Autodesk Inventor part; units mm, degrees
ref_plane "YZ Plane" through (0, 0, 0) normal (1, 0, 0) x (0, 1, 0)
ref_plane "XZ Plane" through (0, 0, 0) normal (0, 1, 0) x (-1, 0, 0)
ref_plane "XY Plane" through (0, 0, 0) normal (0, 0, 1) x (1, 0, 0)
sketch "Skizze1" plane through (0, 0, 0) normal (0, 0, 1) x (1, 0, 0)
  line L0 (-20, 20) -> (20, 20)
  line L1 (20, 20) -> (20, -20)
  line L2 (20, -20) -> (-20, -20)
  line L3 (-20, -20) -> (-20, 20)
  line L4 (0, 20) -> (0, -20)
  line L5 (-20, 0) -> (20, 0)
  point P0 (0, 0)
  point P1 (0, 0)
  point P2 (-20, 0)
  point P3 (0, 0)
  point P4 (20, 0)
  dimension "d1" = 40
  dimension "d2" = 40
extrude "Extrusion1" add sketch "Skizze1" along normal blind 0.5
sketch "Skizze2" plane through (0, 0, 0.5) normal (0, 0, 1) x (1, 0, 0)
  line L0 (-20, -20) -> (20, -20)
  line L1 (-4.5, -20) -> (4.5, -20)
  line L2 (4.5, -20) -> (4.5, -25)
  line L3 (4.5, -25) -> (-4.5, -25)
  line L4 (-4.5, -25) -> (-4.5, -20)
  line L5 (0, -20) -> (0, -25)
  point P0 (0, 0)
  dimension "d5" = 5
  dimension "d6" = 9
extrude "Extrusion2" add sketch "Skizze2" along normal blind 7 and the other way blind 0.5
sketch "Skizze3" plane through (-4.5, -20, 0.5) normal (0, 1, 0) x (1, 0, 0)
  line L0 (0, -7) -> (0, 0)
  line L1 (9, 0.5) -> (0, 0.5)
  line L2 (0, -7) -> (9, 0.5)
  line L3 (9, 0.5) -> (9, -6.5)
  line L4 (9, -6.5) -> (0, 0)
  circle A0 centre (4.5, -3.25) radius 0.5388
  point P0 (4.5, 0.5)
  point P1 (0, 0.5)
hole "Bohrung1" at (0, -20, 3.75) direction (0, -1, 0) diameter 2.459 end through all
equation "\"d2\" = d1"
properties part number "basicdifuser"
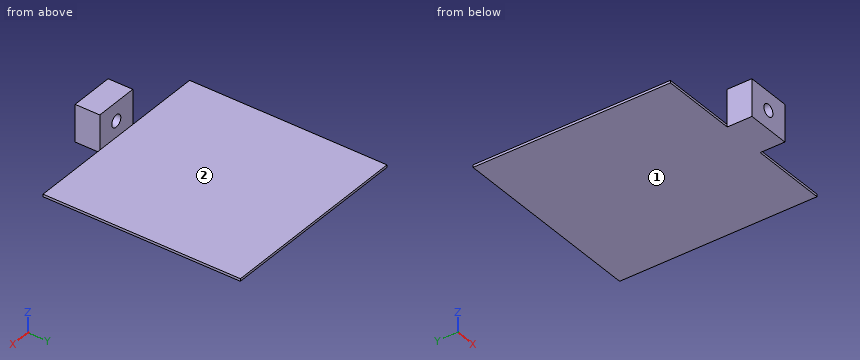
For this review, take the finished solid that the model builds, in its own axes (mm). Face numbers are marked on the shaded views. A direction names the side the tool comes from. Coordinates: 2 decimals unless noted, no trailing zeros. Order: outer loops, then holes, each group sorted by start corner. A loop starts at its lowest first (then second) coordinate and runs counter-clockwise, first axis right, second up. Notation, with made-up numbers: (-22, 44) - (18, 44) arc R12 ccw to (18, 59) - close; hole circle Ø5 at (2, 78). An arc over 180 degrees is marked (long way). Use one line per item in the form item = value.
Q1. For the marked faces 1 and 2, list the 3-axis set-ups (+Z, -Z, +X, -X, +Y, -Y) from which the entire face can be reached by the end or side of a thin tool; tool diameter is ignored.
Checked values:
face_1 = -Z, +X, -X, +Y, -Y
face_2 = +Z, +X, -X, +Y
Q2. Consider section B-B (x = 0). Give the boundary of the cut face in (y, z), then the cut area to 3 significant figures.
Checked values:
outline = (-25, 0) - (20, 0) - (20, 0.5) - (-20, 0.5) - (-20, 2.52) - (-25, 2.52) - close; (-25, 4.98) - (-20, 4.98) - (-20, 7.5) - (-25, 7.5) - close
area = 45.2 mm2
Q3. For P1, Ø3, axis at x = 3.5, y = -10.5, coming from the +Z side; P2, Ø2.5, axis at y = -22, z = 4.5, coming from the -X side; P3, Ø2, axis at x = 0, z = 3.75, coming from the -Y side, all flat-tipped, find the tip position at first contact; note any pin that passes through.
Checked values:
P1 = 0.5
P2 = -4.5
P3 = through
Q4. Consider section A-A (z = 3.75). Give the boundary of the cut face in (x, y).
Checked values:
outline = (-4.5, -25) - (-1.23, -25) - (-1.23, -20) - (-4.5, -20) - close; (1.23, -25) - (4.5, -25) - (4.5, -20) - (1.23, -20) - close
Q5. Consider section C-C (y = -13.5). Give the boundary of the cut face in (x, z).
Checked values:
outline = (-20, 0) - (20, 0) - (20, 0.5) - (-20, 0.5) - close
Q6. For probe 1 along X at (y, z) = (-22.5, 3.75); probe 2 along Z at (x, y) = (0, -21.65); probe 3 along Y at (x, z) = (1, 5.5), list the stretches that pass through material, from the lowest coordinate up. Write a range as from..to.
Checked values:
probe_1 = -4.5..-1.23, 1.23..4.5
probe_2 = 0..2.52, 4.98..7.5
probe_3 = -25..-20
